```python
from build123d import *

# Parameters (mm, degrees)
SKETCH3_R                    = 3
CUT_EXTRUDE2_DEPTH           = 10
SKETCH4_R                    = 5
CUT_EXTRUDE3_DEPTH           = 15
CUT_EXTRUDE_THIN2_DEPTH      = 10
CUT_EXTRUDE_THIN2_DEPTH_BACK = 10
SKETCH5_W                    = 45
SKETCH5_H                    = 37
SKETCH5_W_2                  = 25
SKETCH5_H_2                  = 17


with BuildPart() as part:
    # Sketch1 → Revolve3 (revolve)
    with BuildSketch(Plane.XY, mode=Mode.PRIVATE) as revolve3_sk:
        with BuildLine():
            Line((30, -5), (30, 0))
            Line((30, 0), (5, 0))
            ThreePointArc((5, 0), (0, -5), (-5, 0))
            Line((-5, 0), (-10, 0))
            ThreePointArc((-10, 0), (-2.588190451, -9.659258263), (8.660254038, -5))
            Line((8.660254038, -5), (30, -5))
        make_face()
    revolve(revolve3_sk.sketch.rotate(Axis((-13.11573237, 0, 0), (1, 0, 0)), 270), axis=Axis((-13.11573237, 0, 0), (1, 0, 0)))

    # Sketch3 → Cut-Extrude2 (cut)
    with BuildSketch(Plane(origin=(30, 0, 0), x_dir=(0, 0, -1), z_dir=(1, 0, 0))):
        Circle(SKETCH3_R)
    extrude(amount=-CUT_EXTRUDE2_DEPTH, mode=Mode.SUBTRACT)

    # Sketch2 → Cut-Revolve1 (revolve, cut)
    with BuildSketch(Plane.XY):
        with BuildLine():
            Line((-6.5, 0), (6.5, 0))
            ThreePointArc((6.5, 0), (0, -6.5), (-6.5, 0))
        make_face()
    revolve(axis=Axis((-6.5, 0, 0), (1, 0, 0)), mode=Mode.SUBTRACT)

    # Sketch4 → Cut-Extrude3 (cut, symmetric)
    with BuildSketch(Plane(origin=(0, 0, 0), x_dir=(1, 0, 0), z_dir=(0, 1, 0))):
        with Locations(Location((0, 0, 0), (0, 0, 270))):
            Circle(SKETCH4_R)
    extrude(amount=CUT_EXTRUDE3_DEPTH, both=True, mode=Mode.SUBTRACT)

    # Sketch5 → Cut-Extrude-Thin2 (cut, two sides: drawn at the far end of the back side and taken through both)
    with BuildSketch(Plane(origin=(0, 0, 0), x_dir=(0, 0, -1), z_dir=(1, 0, 0)).offset(-CUT_EXTRUDE_THIN2_DEPTH_BACK)):
        Rectangle(SKETCH5_W, SKETCH5_H)
        Rectangle(SKETCH5_W_2, SKETCH5_H_2, mode=Mode.SUBTRACT)
    extrude(amount=CUT_EXTRUDE_THIN2_DEPTH + CUT_EXTRUDE_THIN2_DEPTH_BACK, mode=Mode.SUBTRACT)


solid = part.part
```
For this review, take the finished solid that the model builds, in its own axes (mm). Give positions to 0.01 mm unless a question says otherwise; leave off trailing zeros. Write each loop counter-clockwise with the first axis right and the second up, starting at its lowest first coordinate (ties: lowest second). Pieces come first, ordered by that corner, then holes.
Item 1: Take a section at B-B (z = 0). Give the boundary of the cut face in (x, y), and give its area (3 significant figures).
Item 2: Wall thickness on probe 1 along Y at (x, z) = (26.5, 0); probe 2 along X at (y, z) = (-3.5, -6.75); probe 3 along Y at (x, z) = (21, 2.25): over which ranges is each line inside the solid? List them lowest first.
Item 3: Take a section at A-A (x = 0). Give the boundary of the cut face in (y, z).
Item 4: Take a section at C-C (y = 0). Give the boundary of the cut face in (x, z).
Item 5: Insertion check: P1, Ø12, axis at x = 22, z = 4.5, coming from the +Y side; P2, Ø3, axis at x = -2, y = 0, coming from the -Z side; P3, Ø6, axis at y = 4.5, z = 0, coming from the -X side. Each pin has a flat end and moves straight along its axis. Give the tip position at first contact, or say it passes through.
Item 6: Take a section at D-D (x = 6). Give the boundary of the cut face in (y, z).
Item 7: The part is to be moulded in two halves that separate along X. For faces 1 (the face through (-4.88, -6.3, -1.08)), 2 (the face through (19.48, 4.88, -1.08)), 3 (the face through (30, 3.3, -0.1)), 4 (the face through (-4.88, 6.36, -1.08)), say which applies: +X half, -X half, draft (parallel to the pull), parting line (faces both ways), or undercut.
Established:
1. outline: (-5.27, -8.5) - (-5, -8.5) - (-5, -4.15) arc R6.5 cw to (-5, 4.15) - (-5, 8.5) - (-5.27, 8.5) arc R10 ccw to start; (5, -8.5) - (5.27, -8.5) arc R10 ccw to (8.66, -5) - (30, -5) - (30, -3) - (20, -3) - (20, 3) - (30, 3) - (30, 5) - (8.66, 5) arc R10 ccw to (5.27, 8.5) - (5, 8.5) - (5, 4.15) arc R6.5 cw to (5, -4.15) - close
1. area: 250 mm2
2. probe 1: y = -5 to -3, 3 to 5
2. probe 2: x = -6.5 to 6.5
2. probe 3: y = -4.47 to -1.98, 1.98 to 4.47
3. outline: (-8.5, -5.27) arc R10 ccw to (8.5, -5.27) - (8.5, -5) - (4.15, -5) arc R6.5 cw to (-4.15, -5) - (-8.5, -5) - close; (-8.5, 5) - (-4.15, 5) arc R6.5 cw to (4.15, 5) - (8.5, 5) - (8.5, 5.27) arc R10 ccw to (-8.5, 5.27) - close
4. outline: (8.66, -5) - (30, -5) - (30, -3) - (20, -3) - (20, 3) - (30, 3) - (30, 5) - (8.66, 5) arc R10 ccw (long way) to start; hole circle Ø13 at (0, 0)
5. P1: stops at y = 5
5. P2: stops at z = -9.99
5. P3: stops at x = -9.89
6. outline: circle Ø16 at (0, 0); hole circle Ø5 at (0, 0)
7. face 1: undercut
7. face 2: draft
7. face 3: +X half
7. face 4: undercut
